Work out the finished part from the listing and answer in its coordinate system (mm). Face numbers are marked on the shaded views. A direction names the side the tool comes from. Round coordinates to 2 decimals unless told otherwise and drop trailing zeros. Loops run counter-clockwise (first coordinate to the right, second up) from the corner with the lowest first, then second, coordinate; pieces in that order, holes last. Notation, with made-up numbers: (13.25, -32.75) - (65.25, -32.75) arc R9 ccw to (65.25, -15.75) - close; hole circle Ø11 at (31, 66). An arc over 180 degrees is marked (long way). Answer as CSV lines item,"result". Start each with the question number.
Q1. Each of these flat-tipped pins is pushed along its axis until it touches: pin 1 Ø4 at (x, z) = (58, -1.5) entering from +Y; pin 2 Ø3 at (x, y) = (70, 16.5) entering from +Z; pin 3 Ø3 at (x, y) = (70.5, 17) entering from -Z; pin 4 Ø9 at (x, z) = (61.595, -14.605) entering from -Y. Where does it stop, or does it pass through?
Q2. For the marked faces 1 and 2, determine the directions among +Z, -Z, +X, -X, +Y, -Y from which every point of the face is accessible in a straight line to the end or side of a thin tool.
Q3. Section C-C on y = 11.75 is taken. Write down the section's boundary in (x, z).
Q4. Straight lines are drawn through the part: L1, parallel to Y at x = 34, z = 1; L2, parallel to X at y = 9, z = -2; L3, parallel to X at y = 2, z = 4. For each, find the intervals that lie inside material, in ascending order. Write a range as [from, to].
Q5. Section B-B on x = -18 is taken. Write down the section's boundary in (y, z).
Q6. Section A-A on z = 0 is taken. Write down the section's boundary in (x, y).
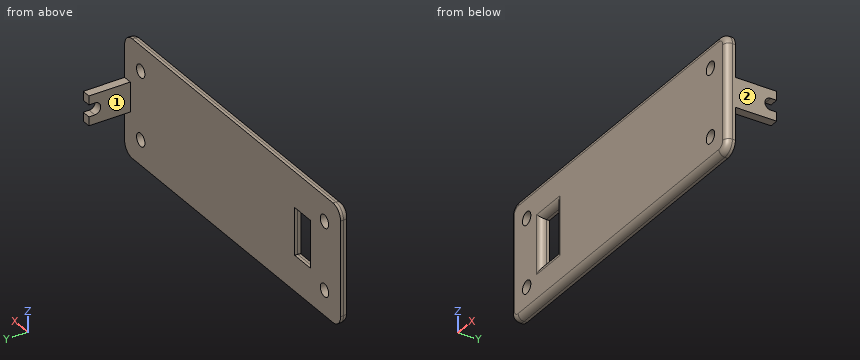
```python
from build123d import *

# Parameters (mm, degrees)
SKETCH1_W           = 144.78
SKETCH1_H           = 50.8
BOSS_EXTRUDE1_DEPTH = 3.81
SKETCH2_W           = 3.81
SKETCH2_H           = 12.7
BOSS_EXTRUDE2_DEPTH = 17.78
CUT_EXTRUDE1_REACH  = 146.78
SKETCH4_W           = 10.668
SKETCH4_H           = 20.32
CUT_EXTRUDE2_DEPTH  = 22.59
SKETCH5_R           = 2.794
CUT_EXTRUDE3_DEPTH  = 22.59
FILLET3_R           = 5.08
FILLET4_R           = 2.54


with BuildPart() as part:
    # Sketch1 → Boss-Extrude1 (new body)
    with BuildSketch(Plane(origin=(0, 0, 0), x_dir=(1, 0, 0), z_dir=(0, 1, 0))):
        Rectangle(SKETCH1_W, SKETCH1_H)
    extrude(amount=BOSS_EXTRUDE1_DEPTH)

    # Sketch2 → Boss-Extrude2 (add)
    with BuildSketch(Plane(origin=(0, 3.81, 0), x_dir=(1, 0, 0), z_dir=(0, 1, 0))):
        with Locations((70.485, 0)):
            Rectangle(SKETCH2_W, SKETCH2_H)
    extrude(amount=BOSS_EXTRUDE2_DEPTH)

    # Sketch3 → Cut-Extrude1 (cut, up to next)
    with BuildSketch(Plane(origin=(72.39, 0, 0), x_dir=(0, 0, -1), z_dir=(1, 0, 0)), mode=Mode.PRIVATE) as cut_extrude1_sk1:
        with BuildLine():
            Line((-2.54, 21.59), (2.54, 21.59))
            Line((2.54, 21.59), (2.54, 19.05))
            ThreePointArc((2.54, 19.05), (0, 16.51), (-2.54, 19.05))
            Line((-2.54, 19.05), (-2.54, 21.59))
        make_face()
    cut_extrude1_tool1 = extrude(cut_extrude1_sk1.sketch, amount=-CUT_EXTRUDE1_REACH, mode=Mode.PRIVATE) & part.part
    add(cut_extrude1_tool1.solids().sort_by_distance((72.39, 19.287109, 0))[0], mode=Mode.SUBTRACT)

    # Sketch4 → Cut-Extrude2 (cut, through all)
    with BuildSketch(Plane.XZ):
        with Locations((-46.976, 0)):
            Rectangle(SKETCH4_W, SKETCH4_H)
    extrude(amount=-CUT_EXTRUDE2_DEPTH, mode=Mode.SUBTRACT)

    # Sketch5 → Cut-Extrude3 (cut, through all)
    with BuildSketch(Plane.XZ):
        with Locations((61.595, -14.605)):
            Circle(SKETCH5_R)
        with Locations((61.595, 14.605)):
            Circle(SKETCH5_R)
        with Locations((-61.595, 14.605)):
            Circle(SKETCH5_R)
        with Locations((-61.595, -14.605)):
            Circle(SKETCH5_R)
    extrude(amount=-CUT_EXTRUDE3_DEPTH, mode=Mode.SUBTRACT)

    # Fillet3
    fillet3_edges = [part.edges().sort_by_distance(p)[0] for p in [
        (72.39, 1.905, 25.4),
        (-72.39, 1.905, 25.4),
        (-72.39, 1.905, -25.4),
        (72.39, 1.905, -25.4),
    ]]
    fillet(fillet3_edges, radius=FILLET3_R)

    # Fillet4
    fillet4_edges = [part.edges().sort_by_distance(p)[0] for p in [
        (-52.31, 0, 0),
        (-46.976, 0, -10.16),
        (-41.642, 0, 0),
        (-46.976, 0, 10.16),
        (-72.39, 0, 0),
        (72.39, 0, 0),
        (0, 0, 25.4),
        (0, 0, -25.4),
        (70.902102448, 0, -23.912102448),
        (70.902102448, 0, 23.912102448),
        (-70.902102448, 0, 23.912102448),
        (-70.902102448, 0, -23.912102448),
    ]]
    fillet(fillet4_edges, radius=FILLET4_R)


solid = part.part
```
Findings:
1,pin 1,"stops at y = 3.81"
1,pin 2,"stops at z = 6.35"
1,pin 3,"stops at z = -6.35"
1,pin 4,"stops at y = 0"
2,face 1,"+Z, -Z, -X, +Y"
2,face 2,"+Z, -Z, +X, +Y, -Y"
3,outline,"(68.58, -6.35) - (72.39, -6.35) - (72.39, 6.35) - (68.58, 6.35) - close"
4,L1,"y = [0, 3.81]"
4,L2,"x = [68.58, 72.39]"
4,L3,"x = [-72.33, -52.37], [-41.58, 72.33]"
5,outline,"(0, -22.86) arc R2.54 ccw to (2.54, -25.4) - (3.81, -25.4) - (3.81, 25.4) - (2.54, 25.4) arc R2.54 ccw to (0, 22.86) - close"
6,outline,"(-72.39, 2.54) arc R2.54 ccw to (-69.85, 0) - (-54.85, 0) arc R2.54 ccw to (-52.31, 2.54) - (-52.31, 3.81) - (-72.39, 3.81) - close; (-41.64, 2.54) arc R2.54 ccw to (-39.1, 0) - (69.85, 0) arc R2.54 ccw to (72.39, 2.54) - (72.39, 16.51) - (68.58, 16.51) - (68.58, 3.81) - (-41.64, 3.81) - close"
